from build123d import *

# Parameters (mm, degrees)
CROQUIS1_R              = 9.525
SALIENTE_EXTRUIR1_DEPTH = 50
SALIENTE_EXTRUIR2_START = -16
CROQUIS3_R              = 9.525
SALIENTE_EXTRUIR2_DEPTH = 16
CROQUIS4_R              = 9.525
SALIENTE_EXTRUIR3_DEPTH = 15
CHAFL_N1_SIZE           = 3
CHAFL_N1_SIZE2          = 1.732050808
CROQUIS5_R              = 52.693762875
CROQUIS5_R_2            = 14
CORTAR_EXTRUIR1_DEPTH   = 15
CORTAR_EXTRUIR1_DRAFT   = -51
CROQUIS6_R              = 45.15885801
CROQUIS6_R_2            = 14
CORTAR_EXTRUIR2_DEPTH   = 15
CORTAR_EXTRUIR2_DRAFT   = -50


with BuildPart() as part:
    # Croquis1 → Saliente-Extruir1 (new body)
    with BuildSketch(Plane(origin=(0, 0, 0), x_dir=(1, 0, 0), z_dir=(0, 1, 0))):
        with Locations(Location((0, 0, 0), (0, 0, 270))):
            Circle(CROQUIS1_R)
    extrude(amount=SALIENTE_EXTRUIR1_DEPTH)

    # Croquis3 → Saliente-Extruir2 (add)
    with BuildSketch(Plane(origin=(0, 50, 0), x_dir=(1, 0, 0), z_dir=(0, 1, 0)).offset(SALIENTE_EXTRUIR2_START)):
        Polygon((16.165807537, 0), (8.082903769, 14), (-8.082903769, 14), (-16.165807537, 0), (-8.082903769, -14), (8.082903769, -14), align=None)
        with Locations(Location((0, 0, 0), (0, 0, 270))):
            Circle(CROQUIS3_R, mode=Mode.SUBTRACT)
    extrude(amount=SALIENTE_EXTRUIR2_DEPTH)

    # Croquis4 → Saliente-Extruir3 (add)
    with BuildSketch(Plane(origin=(0, 50, 0), x_dir=(1, 0, 0), z_dir=(0, 1, 0))):
        with Locations(Location((0, 0, 0), (0, 0, 270))):
            Circle(CROQUIS4_R)
    extrude(amount=SALIENTE_EXTRUIR3_DEPTH)

    # Chaflán1
    chafl_n1_edges = [part.edges().sort_by_distance(p)[0] for p in [
        (0, 65, -9.525),
    ]]
    chafl_n1_side = [part.faces().sort_by_distance(p)[0] for p in [
        (0, 57.5, -9.525),
    ]]
    chamfer(chafl_n1_edges, length=CHAFL_N1_SIZE, length2=CHAFL_N1_SIZE2, reference=chafl_n1_side[0])


with BuildPart() as cortar_extruir1_tool:
    # Croquis5 → Cortar-Extruir1 (with draft: the straight prism first)
    with BuildSketch(Plane(origin=(0, 50, 0), x_dir=(1, 0, 0), z_dir=(0, 1, 0))):
        Circle(CROQUIS5_R)
        Circle(CROQUIS5_R_2, mode=Mode.SUBTRACT)
    extrude(amount=-CORTAR_EXTRUIR1_DEPTH)
    # Cortar-Extruir1: the draft: its side faces are tilted about the plane it starts from
    cortar_extruir1_sides = [cortar_extruir1_tool.faces().sort_by_distance(p)[0] for p in [
        (-52.693762875, 42.5, 0),
        (-14, 42.5, 0),
    ]]
    draft(cortar_extruir1_sides, Plane(origin=(0, 50, 0), x_dir=(1, 0, 0), z_dir=(0, 1, 0)), CORTAR_EXTRUIR1_DRAFT)


with BuildPart() as part_1:
    add(part.part)

    # Cortar-Extruir1: cut by cortar_extruir1_tool
    add(cortar_extruir1_tool.part, mode=Mode.SUBTRACT)


with BuildPart() as cortar_extruir2_tool:
    # Croquis6 → Cortar-Extruir2 (with draft: the straight prism first)
    with BuildSketch(Plane.XZ.offset(-34)):
        Circle(CROQUIS6_R)
        Circle(CROQUIS6_R_2, mode=Mode.SUBTRACT)
    extrude(amount=-CORTAR_EXTRUIR2_DEPTH)
    # Cortar-Extruir2: the draft: its side faces are tilted about the plane it starts from
    cortar_extruir2_sides = [cortar_extruir2_tool.faces().sort_by_distance(p)[0] for p in [
        (-45.15885801, 41.5, 0),
        (-14, 41.5, 0),
    ]]
    draft(cortar_extruir2_sides, Plane.XZ.offset(-34), CORTAR_EXTRUIR2_DRAFT)


with BuildPart() as part_2:
    add(part_1.part)

    # Cortar-Extruir2: cut by cortar_extruir2_tool
    add(cortar_extruir2_tool.part, mode=Mode.SUBTRACT)


solid = part_2.part
For this review, take the finished solid that the model builds, in its own axes (mm). A direction names the side the tool comes from. Give positions to 0.01 mm unless a question says otherwise; leave off trailing zeros. Loops run counter-clockwise (first coordinate to the right, second up) from the corner with the lowest first, then second, coordinate; pieces in that order, holes last. Notation, with made-up numbers: M 58.25,85.5 L 101.25,85.5 A22 ccw 101.25,123.5 Z; hole C 65,-14 d1. An arc over 180 degrees is marked long. Answer as a JSON object with one key per item and string values. Group by question number.
Q1. Mouldability with a two-part tool opening along Y and no side actions: class faces 4 (the conical face through (14.516, 34.433, -0.035)), 5 (the flat face through (-3.3, 50, 9.1)), 6 (the flat face through (-12.18, 41.89, 6.9)) as +Y half, -Y half, draft (parallel to the pull), parting line (faces both ways), or undercut.
Q2. Insertion check: P1, Ø4, axis at x = 8.5, y = 49.5, coming from the -Z side; P2, Ø3, axis at x = 10, z = -11, coming from the -Y side; P3, Ø6, axis at y = 39, z = -11, coming from the +X side; P4, Ø2, axis at y = 23.5, z = -0.5, coming from the +X side (3 decimals). Each pin has a flat end and moves straight along its axis. Give the tip position at first contact, or say it passes through.
Q3. Add section A-A on y = 9. Give the boundary of the cut face in (x, z) (3 decimals).
Q4. For probe 1 along Y at (x, z) = (13, 0.25); probe 2 along X at (y, z) = (56.5, -0.5); probe 3 along X at (y, z) = (54.5, -1.25), list the stretches that pass through material, from the lowest coordinate up. Write a range as [from, to].
Q5. Tool access review of faces 1 (the conical face through (-14.52, 49.58, -0.04)), 2 (the cylindrical face through (-5.796, 16.762, -7.559)), 3 (the cylindrical face through (-5.796, 55.916, -7.559)): name each direction out of +Z, -Z, +X, -X, +Y, -Y from which nothing blocks a thin tool from reaching the whole face with its end or side.
Checked values:
{
 "1": {"face 4": "-Y half", "face 5": "+Y half", "face 6": "draft"},
 "2": {"P1": "z = -14", "P2": "y = 34", "P3": "x = 11.55", "P4": "x = 9.525"},
 "3": {"outline": "C 0,0 d19.05"},
 "4": {"probe 1": "[34, 50]", "probe 2": "[-9.51, 9.51]", "probe 3": "[-9.44, 9.44]"},
 "5": {"face 1": "-X, +Y", "face 2": "-Y", "face 3": "+Y"}
}
